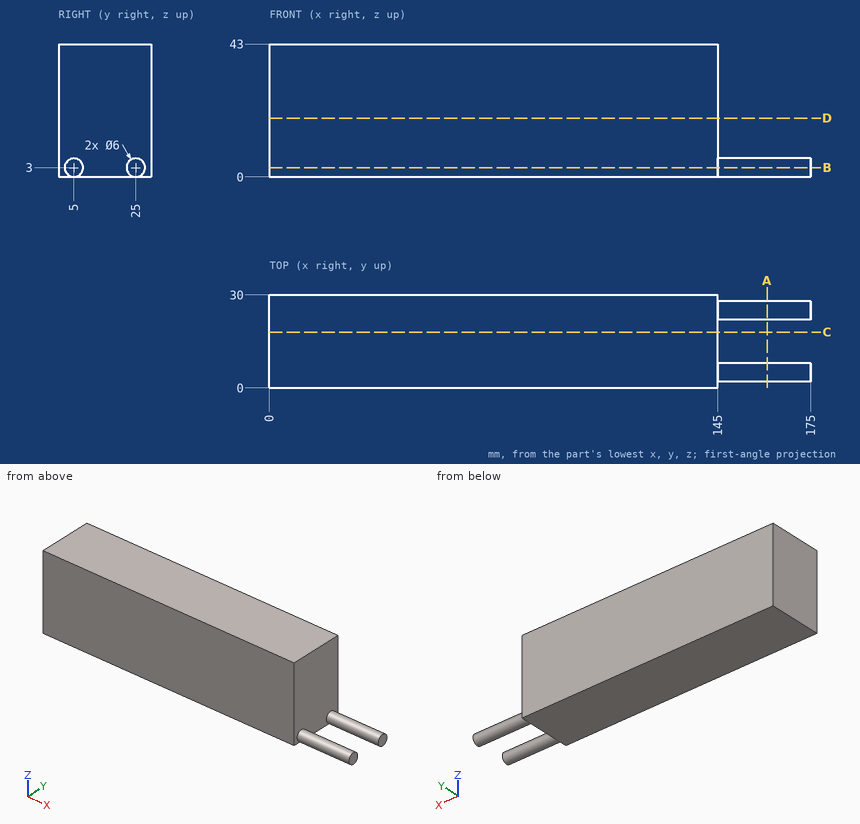
Could you check a few things on this drawing? It's one solid part, dimensions in mm from its lowest x, y, z. Give positions to 0.01 mm unless a question says otherwise; leave off trailing zeros. Order: outer loops, then holes, each group sorted by start corner. A loop starts at its lowest first (then second) coordinate and runs counter-clockwise, first axis right, second up. Notation, with made-up numbers: (24, 82) -> (72, 82) arc R27 ccw to (72, 121) -> close; hole circle Ø3 at (-9.75, -12.5). An arc over 180 degrees is marked (long way). Use CSV: the item, a comma, the result in double quotes. Start each with the question number.
Item 1: Suppose I cut it at A-A (x = 161). List the corners of the cut face in (y, z) for me.
Item 2: Suppose I cut it at B-B (z = 3). List the corners of the cut face in (x, y) for me.
Item 3: I'm going to push a flat-ended pin straight in: P1, Ø10, axis at y = 4, z = 19.5, coming from the +X side. Where does the tip first touch, or does it pass through?
Item 4: Suppose I cut it at C-C (y = 18). List the corners of the cut face in (x, z) for me, and give its area (4 significant figures).
Item 5: Suppose I cut it at D-D (z = 19). List the corners of the cut face in (x, y) for me, and give its area (3 significant figures).
Item 6: If I drill on probe 1 along X at (y, z) = (18.5, 6); probe 2 along Z at (x, y) = (148.5, 22.5), over which ranges is the centre line in solid material (lowest first)? Write a range as [from, to].
Answer block:
1,outline,"circle Ø6 at (5, 3); circle Ø6 at (25, 3)"
2,outline,"(0, 0) -> (145, 0) -> (145, 2) -> (175, 2) -> (175, 8) -> (145, 8) -> (145, 22) -> (175, 22) -> (175, 28) -> (145, 28) -> (145, 30) -> (0, 30) -> close"
3,P1,"stops at x = 145"
4,outline,"(0, 0) -> (145, 0) -> (145, 43) -> (0, 43) -> close"
4,area,"6,235 mm^2"
5,outline,"(0, 0) -> (145, 0) -> (145, 30) -> (0, 30) -> close"
5,area,"4,350 mm^2"
6,probe 1,"x = [0, 145]"
6,probe 2,"z = [1.34, 4.66]"
